Autodesk Inventor part; units mm, degrees
ref_plane "YZ Plane" through (0, 0, 0) normal (1, 0, 0) x (0, 1, 0)
ref_plane "XZ Plane" through (0, 0, 0) normal (0, 1, 0) x (-1, 0, 0)
ref_plane "XY Plane" through (0, 0, 0) normal (0, 0, 1) x (1, 0, 0)
sketch "Sketch1" plane through (0, 0, 0) normal (0, 1, 0) x (-1, 0, 0)
  line L0 (0, 0) -> (-99, 0)
  line L1 (-99, 0) -> (-99, -60)
  line L2 (-99, -60) -> (0, -60)
  line L3 (0, -60) -> (0, 0)
  dimension "d0" = 99
  dimension "d1" = 60
extrude "Extrusion1" add sketch "Sketch1" along normal blind 4
sketch "Sketch3" plane through (0, 4, 0) normal (0, 1, 0) x (1, 0, 0)
  line L0 (99, 60) -> (0, 60) construction
  line L1 (0, 60) -> (0, 0) construction
  line L2 (0, 0) -> (99, 0) construction
  line L3 (99, 0) -> (99, 60) construction
  line L4 (4, 56) -> (95, 56) construction
  line L5 (95, 56) -> (95, 4) construction
  line L6 (95, 4) -> (4, 4) construction
  line L7 (4, 4) -> (4, 56) construction
  line L8 (0, 30) -> (99, 30) construction
  line L9 (49.5, 0) -> (49.5, 60) construction
  line L10 (0, 50) -> (0, 60)
  line L11 (0, 60) -> (13.5, 60)
  line L12 (13.5, 60) -> (13.5, 56)
  line L13 (13.5, 56) -> (4, 56)
  line L14 (4, 56) -> (4, 50)
  line L15 (4, 50) -> (0, 50)
  line L16 (0, 34) -> (4, 34)
  line L17 (4, 34) -> (4, 42)
  line L18 (4, 42) -> (0, 42)
  line L19 (0, 42) -> (0, 34)
  line L20 (45.5, 56) -> (37.5, 56)
  line L21 (37.5, 56) -> (37.5, 60)
  line L22 (37.5, 60) -> (45.5, 60)
  line L23 (45.5, 60) -> (45.5, 56)
  line L24 (29.5, 56) -> (21.5, 56)
  line L25 (21.5, 56) -> (21.5, 60)
  line L26 (21.5, 60) -> (29.5, 60)
  line L27 (29.5, 60) -> (29.5, 56)
  line L28 (0, 10) -> (0, 0)
  line L29 (0, 0) -> (13.5, 0)
  line L30 (13.5, 0) -> (13.5, 4)
  line L31 (13.5, 4) -> (4, 4)
  line L32 (4, 4) -> (4, 10)
  line L33 (4, 10) -> (0, 10)
  line L34 (0, 26) -> (4, 26)
  line L35 (4, 26) -> (4, 18)
  line L36 (4, 18) -> (0, 18)
  line L37 (0, 18) -> (0, 26)
  line L38 (45.5, 4) -> (37.5, 4)
  line L39 (37.5, 4) -> (37.5, 0)
  line L40 (37.5, 0) -> (45.5, 0)
  line L41 (45.5, 0) -> (45.5, 4)
  line L42 (29.5, 4) -> (21.5, 4)
  line L43 (21.5, 4) -> (21.5, 0)
  line L44 (21.5, 0) -> (29.5, 0)
  line L45 (29.5, 0) -> (29.5, 4)
  line L46 (99, 60) -> (99, 0) construction
  line L47 (95, 4) -> (95, 56) construction
  line L48 (99, 50) -> (99, 60)
  line L49 (99, 60) -> (85.5, 60)
  line L50 (85.5, 60) -> (85.5, 56)
  line L51 (85.5, 56) -> (95, 56)
  line L52 (95, 56) -> (95, 50)
  line L53 (95, 50) -> (99, 50)
  line L54 (99, 34) -> (95, 34)
  line L55 (95, 34) -> (95, 42)
  line L56 (95, 42) -> (99, 42)
  line L57 (99, 42) -> (99, 34)
  line L58 (53.5, 56) -> (61.5, 56)
  line L59 (61.5, 56) -> (61.5, 60)
  line L60 (61.5, 60) -> (53.5, 60)
  line L61 (53.5, 60) -> (53.5, 56)
  line L62 (69.5, 56) -> (77.5, 56)
  line L63 (77.5, 56) -> (77.5, 60)
  line L64 (77.5, 60) -> (69.5, 60)
  line L65 (69.5, 60) -> (69.5, 56)
  line L66 (77.5, 4) -> (77.5, 0)
  line L67 (69.5, 4) -> (77.5, 4)
  line L68 (77.5, 0) -> (69.5, 0)
  line L69 (69.5, 0) -> (69.5, 4)
  line L70 (61.5, 4) -> (61.5, 0)
  line L71 (53.5, 0) -> (53.5, 4)
  line L72 (53.5, 4) -> (61.5, 4)
  line L73 (61.5, 0) -> (53.5, 0)
  line L74 (85.5, 0) -> (85.5, 4)
  line L75 (85.5, 4) -> (95, 4)
  line L76 (95, 4) -> (95, 10)
  line L77 (99, 0) -> (85.5, 0)
  line L78 (99, 10) -> (99, 0)
  line L79 (95, 10) -> (99, 10)
  line L80 (95, 18) -> (99, 18)
  line L81 (95, 26) -> (95, 18)
  line L82 (99, 18) -> (99, 26)
  line L83 (99, 26) -> (95, 26)
  dimension "d11" = 4
  dimension "d12" = 8
  dimension "d13" = 4
  dimension "d14" = 8
  dimension "d15" = 8
  dimension "d16" = 4
  dimension "d17" = 8
  dimension "d18" = 8
  dimension "d19" = 8
extrude "Extrusion3" cut sketch "Sketch3" against normal up to surface (4 mm away)
sketch "Sketch5" plane through (0, 4, 0) normal (0, 1, 0) x (1, 0, 0)
  line L0 (77.5, 0) -> (85.5, 0)
  line L1 (99, 42) -> (99, 50)
  line L2 (21.5, 60) -> (13.5, 60)
  line L3 (0, 18) -> (0, 10)
  line L4 (4, 56) -> (95, 56)
  line L5 (95, 56) -> (95, 4)
  line L6 (95, 4) -> (4, 4)
  line L7 (4, 4) -> (4, 56)
  line L8 (91, 52) -> (8, 52)
  line L9 (8, 52) -> (8, 8)
  line L10 (8, 8) -> (91, 8)
  line L11 (91, 8) -> (91, 52)
  line L12 (13.5, 60) -> (13.5, 56)
  line L13 (13.5, 56) -> (4, 56)
  line L14 (4, 56) -> (4, 50)
  line L15 (4, 50) -> (0, 50)
  line L16 (0, 50) -> (0, 42)
  line L17 (0, 42) -> (4, 42)
  line L18 (4, 42) -> (4, 34)
  line L19 (4, 34) -> (0, 34)
  line L20 (0, 34) -> (0, 26)
  line L21 (0, 26) -> (4, 26)
  line L22 (4, 26) -> (4, 18)
  line L23 (4, 18) -> (0, 18)
  line L24 (0, 10) -> (4, 10)
  line L25 (4, 10) -> (4, 4)
  line L26 (4, 4) -> (13.5, 4)
  line L27 (13.5, 4) -> (13.5, 0)
  line L28 (13.5, 0) -> (21.5, 0)
  line L29 (21.5, 0) -> (21.5, 4)
  line L30 (21.5, 4) -> (29.5, 4)
  line L31 (29.5, 4) -> (29.5, 0)
  line L32 (29.5, 0) -> (37.5, 0)
  line L33 (37.5, 0) -> (37.5, 4)
  line L34 (37.5, 4) -> (45.5, 4)
  line L35 (45.5, 4) -> (45.5, 0)
  line L36 (45.5, 0) -> (53.5, 0)
  line L37 (53.5, 0) -> (53.5, 4)
  line L38 (53.5, 4) -> (61.5, 4)
  line L39 (61.5, 4) -> (61.5, 0)
  line L40 (61.5, 0) -> (69.5, 0)
  line L41 (69.5, 0) -> (69.5, 4)
  line L42 (69.5, 4) -> (77.5, 4)
  line L43 (77.5, 4) -> (77.5, 0)
  line L44 (85.5, 0) -> (85.5, 4)
  line L45 (85.5, 4) -> (95, 4)
  line L46 (95, 4) -> (95, 10)
  line L47 (95, 10) -> (99, 10)
  line L48 (99, 10) -> (99, 18)
  line L49 (99, 18) -> (95, 18)
  line L50 (95, 18) -> (95, 26)
  line L51 (95, 26) -> (99, 26)
  line L52 (99, 26) -> (99, 34)
  line L53 (99, 34) -> (95, 34)
  line L54 (95, 34) -> (95, 42)
  line L55 (95, 42) -> (99, 42)
  line L56 (99, 50) -> (95, 50)
  line L57 (95, 50) -> (95, 56)
  line L58 (95, 56) -> (85.5, 56)
  line L59 (85.5, 56) -> (85.5, 60)
  line L60 (85.5, 60) -> (77.5, 60)
  line L61 (77.5, 60) -> (77.5, 56)
  line L62 (77.5, 56) -> (69.5, 56)
  line L63 (69.5, 56) -> (69.5, 60)
  line L64 (69.5, 60) -> (61.5, 60)
  line L65 (61.5, 60) -> (61.5, 56)
  line L66 (61.5, 56) -> (53.5, 56)
  line L67 (53.5, 56) -> (53.5, 60)
  line L68 (53.5, 60) -> (45.5, 60)
  line L69 (45.5, 60) -> (45.5, 56)
  line L70 (45.5, 56) -> (37.5, 56)
  line L71 (37.5, 56) -> (37.5, 60)
  line L72 (37.5, 60) -> (29.5, 60)
  line L73 (29.5, 60) -> (29.5, 56)
  line L74 (29.5, 56) -> (21.5, 56)
  line L75 (21.5, 56) -> (21.5, 60)
  point P0 (0, 0)
  dimension "d22" = 4
  dimension "d23" = 4
extrude "Extrusion4" add sketch "Sketch5" along normal blind 7 contours L6 L7 L4 L5
properties part number "top" material "PBT Plastic Black"
The listing builds one solid part. Answer for the finished solid, in the listing's coordinates (mm). A direction names the side the tool comes from. Coordinates: 2 decimals unless noted, no trailing zeros. Order: outer loops, then holes, each group sorted by start corner. A loop starts at its lowest first (then second) coordinate and runs counter-clockwise, first axis right, second up. Notation, with made-up numbers: M 16.5,-39.5 L 59.5,-39.5 A25 cw 59.5,-21.5 Z; hole C 23.5,-3 d9. An arc over 180 degrees is marked long. Answer as a JSON object with one key per item and string values. Group by question number.
1. Section D-D on z = -7 is taken. Write down the section's boundary in (x, y).
2. Determine the mould class of faces 1 (the flat face through (2, 2, -34)), 2 (the flat face through (34, 2, -60)), 3 (the flat face through (37.5, 2, -2)), 4 (the flat face through (65, 2, 0)) for opening direction Z: released by +Z, released by -Z, zero draft, split by the parting line, or undercut.
3. A tool of negligible diameter and unlimited length cuts with its end or side. For faces 5 (the flat face through (77.5, 2, -58)), 6 (the flat face through (50, 4, -2)), 7 (the flat face through (13.5, 2, -58)), 8 (the flat face through (2, 4, -46)), 9 (the flat face through (82, 4, -58)), from which of +Z, -Z, +X, -X, +Y, -Y can it reach the whole face along a straight path? Write none if from no direction.
4. Straight lines are drawn through the part: line 1 (Z direction, x = 66, y = 7.5); line 2 (X direction, y = 9.5, z = -51.5); line 3 (Y direction, x = 45.5, z = -24). For each, find the intervals that lie inside material, in ascending order.
5. Section C-C on x = 76.5 is taken. Write down the section's boundary in (y, z), then the cut area to 3 significant figures.
6. Flat-ended cylindrical pins translate along their axes: P1, Ø1.2, axis at y = 3, z = -58, coming from the -X side; P2, Ø3, axis at x = 49.5, z = -1.5, coming from the +Y side; P3, Ø10, axis at x = 40.5, z = -20.5, coming from the -Y side; P4, Ø6, axis at y = 9.5, z = -48.5, coming from the +X side. Find the tip coordinate at first contact, or state that the pin passes through.
7. Section B-B on z = -35 is taken. Write down the section's boundary in (x, y), then the cut area to 3 significant figures.
8. Section A-A on y = 6 is taken. Write down the section's boundary in (x, z).
Values follow:
{
 "1": {"outline": "M 4,0 L 95,0 L 95,11 L 4,11 Z"},
 "2": {"face 1": "undercut", "face 2": "released by -Z", "face 3": "zero draft", "face 4": "released by +Z"},
 "3": {"face 5": "-Z, +Y, -Y", "face 6": "+Z, +X, -X, +Y", "face 7": "-Z, -X, +Y, -Y", "face 8": "+Z, -Z, -X, +Y", "face 9": "-Z, +X, -X, +Y"},
 "4": {"line 1": "-56 to -52, -8 to -4", "line 2": "4 to 8, 91 to 95", "line 3": "0 to 4"},
 "5": {"outline": "M 0,-56 L 11,-56 L 11,-52 L 4,-52 L 4,-8 L 11,-8 L 11,-4 L 0,-4 Z", "area": "264 mm2"},
 "6": {"P1": "x = 13.5", "P2": "y = 4", "P3": "y = 0", "P4": "x = 95"},
 "7": {"outline": "M 4,0 L 95,0 L 95,11 L 91,11 L 91,4 L 8,4 L 8,11 L 4,11 Z", "area": "420 mm2"},
 "8": {"outline": "M 4,-56 L 95,-56 L 95,-4 L 4,-4 Z; hole M 8,-52 L 91,-52 L 91,-8 L 8,-8 Z"}
}
